from build123d import *

# Parameters (mm, degrees)
SKETCH2_R      = 38.092749534
EXTRUDE1_DEPTH = 25.4
SKETCH3_R      = 37.09091208
EXTRUDE2_DEPTH = 6.35
CHAMFER1_SIZE  = 6.35
EXTRUDE7_START = -6.35
SKETCH10_R     = 47.61774957
SKETCH10_R_2   = 38.092749534
EXTRUDE7_DEPTH = 3.175
FILLET1_R      = 3.175
FILLET2_R      = 0.762


with BuildPart() as part:
    # Sketch2 → Extrude1 (new body)
    with BuildSketch(Plane.XY):
        with Locations((332.784130452, 254.345130463)):
            Circle(SKETCH2_R)
    extrude(amount=-EXTRUDE1_DEPTH)

    # Sketch3 → Extrude2 (cut)
    with BuildSketch(Plane.XY):
        with Locations((332.784130452, 254.345130463)):
            Circle(SKETCH3_R)
    extrude(amount=-EXTRUDE2_DEPTH, mode=Mode.SUBTRACT)

    # Chamfer1
    chamfer1_edges = [part.edges().sort_by_distance(p)[0] for p in [
        (295.693218372, 254.345130463, -6.35),
    ]]
    chamfer(chamfer1_edges, length=CHAMFER1_SIZE - 0.0001)  # a hair under: the kernel refuses the full size

    # Sketch10 → Extrude7 (add)
    with BuildSketch(Plane.XY.offset(EXTRUDE7_START)):
        with Locations((332.784130452, 254.345130463)):
            Circle(SKETCH10_R)
        with Locations((332.784130452, 254.345130463)):
            Circle(SKETCH10_R_2, mode=Mode.SUBTRACT)
    extrude(amount=-EXTRUDE7_DEPTH)

    # Fillet1
    fillet1_edges = [part.edges().sort_by_distance(p)[0] for p in [
        (294.691380918, 254.345130463, -6.35),
    ]]
    fillet(fillet1_edges, radius=FILLET1_R)

    # Fillet2
    fillet2_edges = [part.edges().sort_by_distance(p)[0] for p in [
        (285.166380882, 254.345130463, -6.35),
    ]]
    fillet(fillet2_edges, radius=FILLET2_R)


solid = part.part
Can you work these out from the model? Positions are in its coordinate system, mm. A direction names the side the tool comes from. Give positions to 0.01 mm unless a question says otherwise; leave off trailing zeros. Loops run counter-clockwise (first coordinate to the right, second up) from the corner with the lowest first, then second, coordinate; pieces in that order, holes last. Notation, with made-up numbers: M 19.25,69 L 52.25,69 A23 ccw 52.25,80 Z; hole C -5,39 d10. An arc over 180 degrees is marked long. One line per item, written item: value.
1) Imagine slicing it at A-A on z = -2. Write out the boundary of the cut face in (x, y).
Geometry check:
outline: C 332.78,254.35 d76.19; hole C 332.78,254.35 d70.18
2) Please list where these lines run through material, in increasing order: line 1 (Z direction, x = 336, y = 257.5); line 2 (Z direction, x = 349, y = 295) (3 decimals); line 3 (Y direction, x = 331, z = -2.75).
Geometry check:
line 1: z = -25.4 to -6.35
line 2: z = -9.525 to -6.35
line 3: y = 216.29 to 220.05, 288.64 to 292.4
3) On a 3-axis mill with a long thin cutter (end or side, diameter ignored), from which of +Z, -Z, +X, -X, +Y, -Y can I reach the whole of each face in a straight line? I mean faces 1 (the face through (311, 286, -9.525)), 2 (the face through (369.118, 265.787, -1.565)), 3 (the face through (369.3, 246.1, 0)). Say none if no direction works.
Geometry check:
face 1: -Z
face 2: +Z
face 3: +Z, +X, -X, +Y, -Y
4) Imagine slicing it at B-B on z = -17. Write out the boundary of the cut face in (x, y).
Geometry check:
outline: C 332.78,254.35 d76.19
5) Thinking about a two-plate mould opening in Y: for faces 4 (the face through (332.6, 212.9, -6.35)), 5 (the face through (369.118, 265.787, -17.351)), 6 (the face through (332, 255, -6.35)), 7 (the face through (326.053, 224.034, -6.042)), which applies, +Y half, -Y half, draft (parallel to the pull), parting line (faces both ways), or undercut?
Geometry check:
face 4: draft
face 5: parting line
face 6: undercut
face 7: undercut
6) I'm going to push flat-ended pins straight in: pin 1 (3 mm diameter, centred on x = 309.5, z = -19, fed in from +Y); pin 2 (3 mm diameter, centred on x = 355, z = -16, fed in from -Y); pin 3 (5 mm diameter, centred on x = 339.5, y = 230, fed in from +Z). Where does each tip first touch, or does it pass through?
Geometry check:
pin 1: stops at y = 285.59
pin 2: stops at y = 222.38
pin 3: stops at z = -6.35
